Job drawing, mm, ordinate dimensions from the low corner. One solid piece. A direction names the side the tool comes from. Round coordinates to 2 decimals unless told otherwise and drop trailing zeros. Order: outer loops, then holes, each group sorted by start corner. A loop starts at its lowest first (then second) coordinate and runs counter-clockwise, first axis right, second up. Notation, with made-up numbers: (-1.75, 46.25) -> (12.25, 46.25) arc R11 cw to (12.25, 52.25) -> close; hole circle Ø4 at (14, 9.5). An arc over 180 degrees is marked (long way). Use CSV: the item, a comma, the result in double quotes.
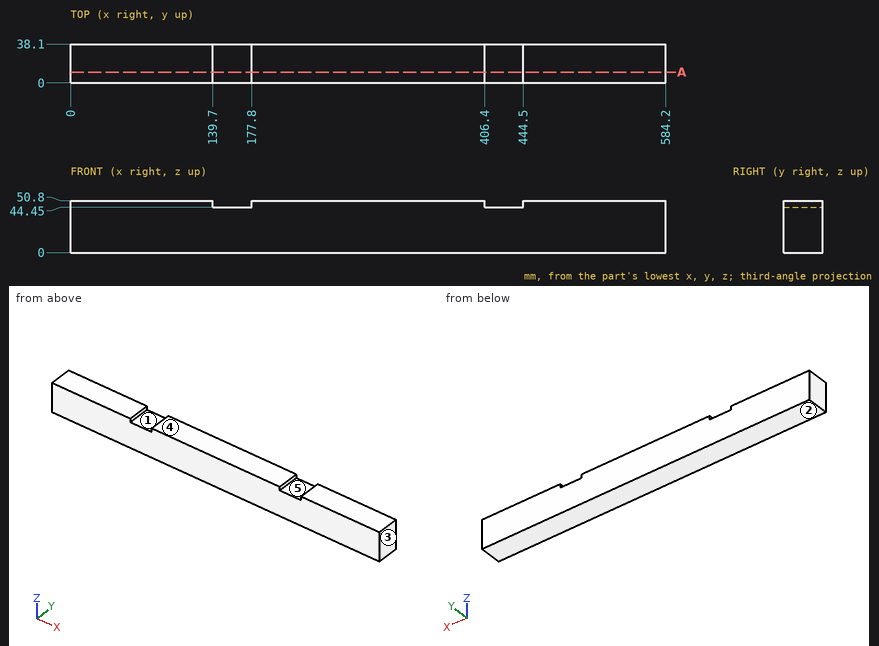
(1) Drop a flat-ended pin along its axis: P1, Ø11.5, axis at x = 159, y = 17, coming from the +Z side. Give the stop position or say it passes through.
Reply:
P1,"z = 44.45"
(2) Probe probe 1 along X at (y, z) = (14, 44.5); probe 2 along Z at (x, y) = (414, 22). List the from-to ranges inside material, lowest first. Write a range as [from, to].
Reply:
probe 1,"[0, 139.7], [177.8, 406.4], [444.5, 584.2]"
probe 2,"[0, 44.45]"
(3) Which spindle directions (+Z, -Z, +X, -X, +Y, -Y) get a long thin tool onto all of the face, cutting with end or side? Do the marked faces 1 and 2. Say none if no direction does.
Reply:
face 1,"+Z, +Y, -Y"
face 2,"-Z, +X, -X, +Y, -Y"
(4) Pull direction X, two halves, no side cores. Call the marked faces 3, 4 and 5: released by +X, released by -X, zero draft, split by the parting line, or undercut.
Reply:
face 3,"released by +X"
face 4,"zero draft"
face 5,"undercut"
(5) Cut at A-A, the plane y = 10.5. Give the cut face in (x, z), then the cut area to 3 significant figures.
Reply:
outline,"(0, 0) -> (584.2, 0) -> (584.2, 50.8) -> (444.5, 50.8) -> (444.5, 44.45) -> (406.4, 44.45) -> (406.4, 50.8) -> (177.8, 50.8) -> (177.8, 44.45) -> (139.7, 44.45) -> (139.7, 50.8) -> (0, 50.8) -> close"
area,"29,200 mm2"
